from build123d import *

# Parameters (mm, degrees)
SKETCH_1_W          = 123
SKETCH_1_H          = 90
EXTRUDE_1_DEPTH     = 14
SKETCH_2_W          = 120
SKETCH_2_H          = 87
CUT_EXTRUDE_1_DEPTH = 12.5
SKETCH_3_W          = 12.5
SKETCH_3_H          = 16
EXTRUDE_2_DEPTH     = 4
SKETCH_4_R          = 4
EXTRUDE_3_DEPTH     = 8.5
SKETCH_5_R          = 3
CUT_EXTRUDE_2_DEPTH = 3
SKETCH_6_R          = 1.6
CUT_EXTRUDE_3_DEPTH = 11
SKETCH_7_R          = 2.6
CUT_EXTRUDE_4_DEPTH = 1.5
SKETCH_8_W          = 22.2
SKETCH_8_H          = 7
SKETCH_8_W_2        = 12
SKETCH_8_H_2        = 6.7
CUT_EXTRUDE_5_DEPTH = 1.5
SKETCH_9_R          = 1.6
CUT_EXTRUDE_6_DEPTH = 4


with BuildPart() as part:
    # Эскиз1 → Бобышка-Вытянуть1 (new body)
    with BuildSketch(Plane(origin=(0, 0, 0), x_dir=(1, 0, 0), z_dir=(0, 1, 0))):
        Rectangle(SKETCH_1_W, SKETCH_1_H)
    extrude(amount=EXTRUDE_1_DEPTH)

    # Эскиз2 → Вырез-Вытянуть1 (cut)
    with BuildSketch(Plane(origin=(0, 14, 0), x_dir=(1, 0, 0), z_dir=(0, 1, 0))):
        Rectangle(SKETCH_2_W, SKETCH_2_H)
    extrude(amount=-CUT_EXTRUDE_1_DEPTH, mode=Mode.SUBTRACT)

    # Эскиз3 → Бобышка-Вытянуть2 (add)
    with BuildSketch(Plane(origin=(0, 1.5, 0), x_dir=(1, 0, 0), z_dir=(0, 1, 0))):
        with Locations((-55.25, 37)):
            Rectangle(SKETCH_3_W, SKETCH_3_H)
        with Locations((55.25, 37)):
            Rectangle(SKETCH_3_W, SKETCH_3_H)
        with Locations((55.25, -37)):
            Rectangle(SKETCH_3_W, SKETCH_3_H)
        with Locations((-55.25, -37)):
            Rectangle(SKETCH_3_W, SKETCH_3_H)
    extrude(amount=EXTRUDE_2_DEPTH)

    # Эскиз4 → Бобышка-Вытянуть3 (add)
    with BuildSketch(Plane(origin=(0, 5.5, 0), x_dir=(1, 0, 0), z_dir=(0, 1, 0))):
        with Locations((-57, 41)):
            Circle(SKETCH_4_R)
        with Locations((57, 41)):
            Circle(SKETCH_4_R)
        with Locations((57, -41)):
            Circle(SKETCH_4_R)
        with Locations((-57, -41)):
            Circle(SKETCH_4_R)
    extrude(amount=EXTRUDE_3_DEPTH)

    # Эскиз5 → Вырез-Вытянуть2 (cut)
    with BuildSketch(Plane(origin=(0, 0, 0), x_dir=(1, 0, 0), z_dir=(0, 1, 0))):
        with Locations(Location((-57, 41, 0), (0, 0, 270))):
            Circle(SKETCH_5_R)
        with Locations(Location((57, 41, 0), (0, 0, 270))):
            Circle(SKETCH_5_R)
        with Locations(Location((57, -41, 0), (0, 0, 270))):
            Circle(SKETCH_5_R)
        with Locations(Location((-57, -41, 0), (0, 0, 270))):
            Circle(SKETCH_5_R)
    extrude(amount=CUT_EXTRUDE_2_DEPTH, mode=Mode.SUBTRACT)

    # Эскиз6 → Вырез-Вытянуть3 (cut)
    with BuildSketch(Plane(origin=(0, 14, 0), x_dir=(1, 0, 0), z_dir=(0, 1, 0))):
        with Locations(Location((-57, 41, 0), (0, 0, 270))):
            Circle(SKETCH_6_R)
        with Locations(Location((57, 41, 0), (0, 0, 270))):
            Circle(SKETCH_6_R)
        with Locations(Location((57, -41, 0), (0, 0, 270))):
            Circle(SKETCH_6_R)
        with Locations(Location((-57, -41, 0), (0, 0, 270))):
            Circle(SKETCH_6_R)
    extrude(amount=-CUT_EXTRUDE_3_DEPTH, mode=Mode.SUBTRACT)

    # Эскиз7 → Вырез-Вытянуть4 (cut)
    with BuildSketch(Plane(origin=(61.5, 0, 0), x_dir=(0, 0, -1), z_dir=(1, 0, 0))):
        with Locations((17, 14)):
            Circle(SKETCH_7_R)
        with Locations((5, 14)):
            Circle(SKETCH_7_R)
    extrude(amount=-CUT_EXTRUDE_4_DEPTH, mode=Mode.SUBTRACT)

    # Эскиз8 → Вырез-Вытянуть5 (cut)
    with BuildSketch(Plane.ZY.offset(61.5)):
        with Locations((0, 10.5)):
            Rectangle(SKETCH_8_W, SKETCH_8_H)
        with Locations((21.5, 10.65)):
            Rectangle(SKETCH_8_W_2, SKETCH_8_H_2)
    extrude(amount=-CUT_EXTRUDE_5_DEPTH, mode=Mode.SUBTRACT)

    # Эскиз9 → Вырез-Вытянуть6 (cut)
    with BuildSketch(Plane(origin=(0, 5.5, 0), x_dir=(-1, 0, 0), z_dir=(0, 1, 0))):
        with Locations(Location((57, 32, 0), (0, 0, 90))):
            Circle(SKETCH_9_R)
        with Locations(Location((57, -32, 0), (0, 0, 90))):
            Circle(SKETCH_9_R)
        with Locations(Location((-57, -32, 0), (0, 0, 90))):
            Circle(SKETCH_9_R)
        with Locations(Location((-57, 32, 0), (0, 0, 90))):
            Circle(SKETCH_9_R)
    extrude(amount=-CUT_EXTRUDE_6_DEPTH, mode=Mode.SUBTRACT)


solid = part.part
Geometry: final body of the model. Coordinates: model frame, mm. A direction names the side the tool comes from. Coordinates: 2 decimals unless noted, no trailing zeros. Order: outer loops, then holes, each group sorted by start corner. A loop starts at its lowest first (then second) coordinate and runs counter-clockwise, first axis right, second up.
(1) Section query A-A (y = 9). Return the cut outline in (x, z).
(2) First-contact query: pin 1 (3 mm diameter, centred on x = 8.5, z = -14.5, fed in from +Y); pin 2 (3.5 mm diameter, centred on x = -57, z = -41, fed in from +Y); pin 3 (3.5 mm diameter, centred on x = -57, z = -41, fed in from -Y); pin 4 (4 mm diameter, centred on x = -57, z = 32, fed in from +Y). Flat tips, straight axial feed; report the tip coordinate or a pass-through.
(3) Material intervals for probe 1 along X at (y, z) = (9.75, -41); probe 2 along X at (y, z) = (2, -12.5); probe 3 along Z at (x, y) = (7.5, 3.5), sorted ascending.
(4) Access query for faces 3 (the face through (54, 3, -29)), 4 (the face through (60.8, 11.4, -16.9)), 5 (the face through (-1, 7, 45)). Directions: +Z, -Z, +X, -X, +Y, -Y. A direction counts if a zero-diameter tool reaches every point of the face in a straight line with its end or side. Return the directions, or none.
(5) Section query B-B (z = 41). Return the cut outline in (x, y), plus the area to 3 significant figures.
(6) Draft query along X for faces 1 (the face through (0, 14, 44)), 2 (the face through (-57, 1.5, 32)). Return one class per face: pulls with the +X half, pulls with the -X half, needs draft (parallel to the pull), parting line crosses it, or undercut.
(7) Section query D-D (x = 39). Return the cut outline in (y, z).
(8) Section query C-C (z = 21). Return the cut outline in (x, y), plus the area to 3 significant figures.
Solution:
1. outline: (-61.5, -45) - (61.5, -45) - (61.5, 45) - (-61.5, 45) - (-61.5, 27.5) - (-60, 27.5) - (-60, 38.35) arc R4 ccw to (-53.88, 43.5) - (53.88, 43.5) arc R4 ccw to (60, 38.35) - (60, -38.35) arc R4 ccw to (53.88, -43.5) - (-53.88, -43.5) arc R4 ccw to (-60, -38.35) - (-60, -11.1) - (-61.5, -11.1) - close; (-61.5, 11.1) - (-60, 11.1) - (-60, 15.5) - (-61.5, 15.5) - close; hole circle Ø3.2 at (-57, -41); hole circle Ø3.2 at (-57, 41); hole circle Ø3.2 at (57, -41); hole circle Ø3.2 at (57, 41)
2. pin 1: stops at y = 1.5
2. pin 2: stops at y = 14
2. pin 3: stops at y = 3
2. pin 4: stops at y = 5.5
3. probe 1: x = -61.5 to -58.6, -55.4 to -53, 53 to 55.4, 58.6 to 61.5
3. probe 2: x = -61.5 to -60, 60 to 61.5
3. probe 3: z = -45 to -43.5, 43.5 to 45
4. face 3: +Y
4. face 4: +X, +Y
4. face 5: +Z, +X, -X, +Y, -Y
5. outline: (-61.5, 0) - (-60, 0) - (-60, 3) - (-58.6, 3) - (-58.6, 14) - (-61.5, 14) - close; (-55.4, 3) - (-54, 3) - (-54, 0) - (54, 0) - (54, 3) - (55.4, 3) - (55.4, 14) - (53, 14) - (53, 5.5) - (49, 5.5) - (49, 1.5) - (-49, 1.5) - (-49, 5.5) - (-53, 5.5) - (-53, 14) - (-55.4, 14) - close; (58.6, 3) - (60, 3) - (60, 0) - (61.5, 0) - (61.5, 14) - (58.6, 14) - close
5. area: 323 mm2
6. face 1: needs draft
6. face 2: undercut
7. outline: (0, -45) - (14, -45) - (14, -43.5) - (1.5, -43.5) - (1.5, 43.5) - (14, 43.5) - (14, 45) - (0, 45) - close
8. outline: (-61.5, 0) - (61.5, 0) - (61.5, 14) - (60, 14) - (60, 1.5) - (-60, 1.5) - (-60, 7.3) - (-61.5, 7.3) - close
8. area: 212 mm2
